```python
from build123d import *

# Parameters (mm, degrees)
F0_W     = 15
F0_H     = 3
F1_DEPTH = 3
F3_DEPTH = 25
F6_COUNT = 6
F8_R     = 3
F9_DEPTH = 3


with BuildPart() as f1:
    # F0 (on Front) → F1 (new body)
    with BuildSketch(Plane.XZ):
        with Locations((9, 38.5)):
            Rectangle(F0_W, F0_H)
        with Locations((9, 31.6)):
            Rectangle(F0_W, F0_H)
        with Locations((9, 24.7)):
            Rectangle(F0_W, F0_H)
        with Locations((9, 17.8)):
            Rectangle(F0_W, F0_H)
        Polygon((0, 40), (0, 0), (1.5, 0), (1.5, 16.3), (1.5, 19.3), (1.5, 23.2), (1.5, 26.2), (1.5, 30.1), (1.5, 33.1), (1.5, 37), (1.5, 40), align=None)
    extrude(amount=F1_DEPTH)

    # F2 (on face) → F3 (cut)
    with BuildSketch(Plane.XZ.offset(3)):
        Polygon((13.405226, 40), (7.321541, 16.3), (20.32141, 16.3), (16.5, 40), align=None)
    extrude(amount=-F3_DEPTH, mode=Mode.SUBTRACT)

    # F4: F1 across plane


with BuildPart() as f1_1:
    add(f1.part)
    add(f1.part.mirror(Plane.YZ))


with BuildPart() as f6_1:
    # F6: instance of F1
    add(f1_1.part.rotate(Axis((0, 13.050985, 0), (0, 1, 0)), 1 * 360 / F6_COUNT))


with BuildPart() as f6_2:
    # F6: instance of F1
    add(f1_1.part.rotate(Axis((0, 13.050985, 0), (0, 1, 0)), 2 * 360 / F6_COUNT))


with BuildPart() as f6_3:
    # F6: instance of F1
    add(f1_1.part.rotate(Axis((0, 13.050985, 0), (0, 1, 0)), 3 * 360 / F6_COUNT))


with BuildPart() as f6_4:
    # F6: instance of F1
    add(f1_1.part.rotate(Axis((0, 13.050985, 0), (0, 1, 0)), 4 * 360 / F6_COUNT))


with BuildPart() as f6_5:
    # F6: instance of F1
    add(f1_1.part.rotate(Axis((0, 13.050985, 0), (0, 1, 0)), 5 * 360 / F6_COUNT))

    # F7: union F1, F6_2, F6_3, F6_4, F6_1
    add(f1_1.part)
    add(f6_2.part)
    add(f6_3.part)
    add(f6_4.part)
    add(f6_1.part)

    # F8 (on face) → F9 (join, through all)
    with BuildSketch(Plane.XZ.offset(3)):
        with BuildLine():
            ThreePointArc((-3.140397, -40), (-1.74903, -47.369217), (4.5, -43.223027))
            ThreePointArc((4.5, -43.223027), (4.14619, -41.473997), (3.140397, -40))
            Line((3.140397, -40), (-3.140397, -40))
        make_face()
        with Locations((0, -43.223027)):
            Circle(F8_R, mode=Mode.SUBTRACT)
    extrude(amount=-F9_DEPTH)


solid = f6_5.part
```
Design review of the part built by this model. Coordinates are the model's own, in mm. A direction names the side the tool comes from. Coordinates: 2 decimals unless noted, no trailing zeros. Loops run counter-clockwise (first coordinate to the right, second up) from the corner with the lowest first, then second, coordinate; pieces in that order, holes last. Notation, with made-up numbers: (82.5, 33) - (141.5, 33) arc R18 ccw to (141.5, 37) - close; hole circle Ø6 at (67, 2.25). An arc over 180 degrees is marked (long way). Use CSV: the item, a comma, the result in double quotes. Start each with the question number.
1) Wall thickness on L1, parallel to Z at x = 0, y = -0.7; L2, parallel to X at y = -2.5, z = -17.5; L3, parallel to Z at x = -27.5, y = -0.85: over which ranges is each line inside the solid? List them lowest first. Write a range as from..to.
2) Consider section A-A on x = 0. Write out the cut boundary in (y, z), then the cut area to 3 significant figures.
3) Tool access review of faces 1 (the flat face through (21.8, -1.5, -25.6)), 2 (the flat face through (-11.931, -1.479, 11.935)): name each direction out of +Z, -Z, +X, -X, +Y, -Y from which nothing blocks a thin tool from reaching the whole face with its end or side.
4) For pin 1 Ø6 at (x, z) = (22.5, -0.5) entering from +Y; pin 2 Ø0.9 at (x, y) = (-6.5, -2) entering from -Z; pin 3 Ø1 at (x, y) = (23.5, -0.5) entering from -Z; pin 4 Ø1 at (x, y) = (19.5, -0.5) entering from +Z, all flat-tipped, find the tip position at first contact; note any pin that passes through.
5) The part is to be moulded in two halves that separate along X. For faces 3 (the flat face through (39.87, -1.52, -7.98)), 4 (the flat face through (-33.012, -1.521, 6.064)), 5 (the flat face through (9.483, -1.521, 24.721)), 6 (the flat face through (-17.63, -1.48, -11.91)), say which applies: +X half, -X half, draft (parallel to the pull), parting line (faces both ways), or undercut.
Geometry says:
1,L1,"-47.72..-46.22, -40.22..40"
1,L2,"-36.08..-24.65, -20.15..-16.69, -7.63..7.63, 16.69..20.15, 24.65..36.08"
1,L3,"-31.18..-26.37, -18.57..-12.57, -4.77..-4.52, 4.52..4.77, 12.57..18.57, 26.37..31.18"
2,outline,"(-3, -47.72) - (0, -47.72) - (0, -46.22) - (-3, -46.22) - close; (-3, -40.22) - (0, -40.22) - (0, 40) - (-3, 40) - close"
2,area,"245 mm^2"
3,face 1,"-Z, +Y, -Y"
3,face 2,"+Y, -Y"
4,pin 1,"y = 0"
4,pin 2,"z = -40"
4,pin 3,"z = -26.36"
4,pin 4,"z = 19.49"
5,face 3,"+X half"
5,face 4,"-X half"
5,face 5,"undercut"
5,face 6,"undercut"
